Verification items for the finished model (mm, model axes). Face numbers are marked on the shaded views. A direction names the side the tool comes from. Coordinates: 2 decimals unless noted, no trailing zeros. Write each loop counter-clockwise with the first axis right and the second up, starting at its lowest first coordinate (ties: lowest second). Pieces come first, ordered by that corner, then holes. Notation, with made-up numbers: (22.5, 53) -> (62.5, 53) arc R10 cw to (62.5, 61) -> close; hole circle Ø1 at (7, -12.5). An arc over 180 degrees is marked (long way). Use CSV: the item, a comma, the result in double quotes.
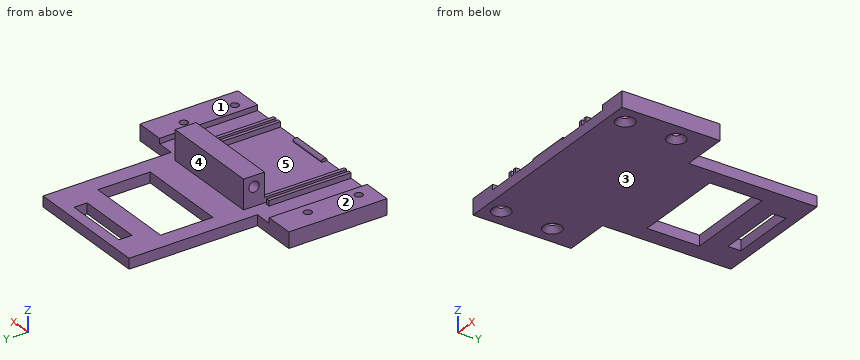
Solid Edge part; units mm, degrees
sketch "Sketch1" plane through (0, 0, 0) normal (0, 0, 1) x (1, 0, 0)
  line L0 (83.1, 37.5) -> (65.55, 37.5)
  line L1 (65.55, 37.5) -> (65.55, 86.5)
  line L2 (65.55, 86.5) -> (17.55, 86.5)
  line L3 (17.55, 86.5) -> (17.55, 37.5)
  line L4 (0, 37.5) -> (17.55, 37.5)
  line L5 (0, 0) -> (0, 37.5)
  line L6 (0, 0) -> (83.1, 0)
  line L7 (83.1, 0) -> (83.1, 37.5)
extrude "Protrusion1" add sketch "Sketch1" along normal blind 4
sketch "Sketch2" plane through (40.5, 43.25, 4) normal (0, 0, 1) x (1, 0, 0)
  line L0 (-29.5, -5.75) -> (-29.5, -43.25)
  line L1 (-29.5, -43.25) -> (-40.5, -43.25)
  line L2 (-40.5, -43.25) -> (-40.5, -5.75)
  line L3 (-40.5, -5.75) -> (-29.5, -5.75)
  line L4 (-20.53, -43.25) -> (-20.53, -11.85)
  line L5 (-20.53, -11.85) -> (-19.23, -11.85)
  line L6 (-19.23, -11.85) -> (-19.23, -43.25)
  line L7 (-19.23, -43.25) -> (-20.53, -43.25)
  line L8 (-16.73, -11.85) -> (-16.73, -43.25)
  line L9 (-16.73, -43.25) -> (-18.03, -43.25)
  line L10 (-18.03, -43.25) -> (-18.03, -11.85)
  line L11 (-18.03, -11.85) -> (-16.73, -11.85)
  line L12 (18.83, -11.85) -> (18.83, -43.25)
  line L13 (18.83, -43.25) -> (20.13, -43.25)
  line L14 (20.13, -43.25) -> (20.13, -11.85)
  line L15 (20.13, -11.85) -> (18.83, -11.85)
  line L16 (22.63, -43.25) -> (22.63, -11.85)
  line L17 (22.63, -11.85) -> (21.33, -11.85)
  line L18 (21.33, -11.85) -> (21.33, -43.25)
  line L19 (21.33, -43.25) -> (22.63, -43.25)
  line L20 (31.6, -5.75) -> (31.6, -43.25)
  line L21 (31.6, -43.25) -> (42.6, -43.25)
  line L22 (42.6, -43.25) -> (42.6, -5.75)
  line L23 (42.6, -5.75) -> (31.6, -5.75)
extrude "ExtrudedProtrusion_2" add sketch "Sketch2" along normal blind 2
sketch "Sketch3" plane through (41.55, 43.25, 4) normal (0, 0, 1) x (1, 0, 0)
  line L0 (-19.08, -11.85) -> (19.08, -11.85)
  line L1 (19.08, -11.85) -> (19.08, -3.85)
  line L2 (19.08, -3.85) -> (-19.08, -3.85)
  line L3 (-19.08, -3.85) -> (-19.08, -11.85)
extrude "ExtrudedProtrusion_3" add sketch "Sketch3" along normal blind 11.2
hole "Hole_1" at (60.63, 35.4, 11.2) direction (-1, 0, 0) diameter 4 depth 6
hole "Hole_2" at (22.47, 35.4, 11.2) direction (1, 0, 0) diameter 4 depth 6
sketch "Sketch4" plane through (41.55, 43.25, 4) normal (0, 0, 1) x (1, 0, 0)
  line L0 (12.5, 34.25) -> (-12.5, 34.25)
  line L1 (-12.5, 34.25) -> (-12.5, 39.25)
  line L2 (-12.5, 39.25) -> (12.5, 39.25)
  line L3 (12.5, 39.25) -> (12.5, 34.25)
  line L4 (-17.5, 26.75) -> (17.5, 26.75)
  line L5 (17.5, 26.75) -> (17.5, 6.75)
  line L6 (17.5, 6.75) -> (-17.5, 6.75)
  line L7 (-17.5, 6.75) -> (-17.5, 26.75)
extrude "Cutout1" cut sketch "Sketch4" against normal through all
hole "Hole_3" at (7, 6, 0) direction (0, 0, 1) diameter 3 end through all countersink diameter 6.94 countersink angle 90
hole "Hole1" at (7, 25.5, 0) direction (0, 0, 1) diameter 3 end through all countersink diameter 6.94 countersink angle 90
hole "Hole2" at (76.1, 6, 0) direction (0, 0, 1) diameter 3 end through all countersink diameter 6.94 countersink angle 90
hole "Hole3" at (76.1, 25.5, 0) direction (0, 0, 1) diameter 3 end through all countersink diameter 6.94 countersink angle 90
sketch "Sketch5" plane through (41.55, 15.7, 4) normal (0, 0, 1) x (1, 0, 0)
  line L0 (-8.0007, -13.7) -> (7.9993, -13.7)
  line L1 (7.9993, -13.7) -> (7.9993, -15.7)
  line L2 (-8.0007, -15.7) -> (7.9993, -15.7)
  line L3 (-8.0007, -13.7) -> (-8.0007, -15.7)
extrude "ExtrudedProtrusion_4" add sketch "Sketch5" along normal blind 1
fillet "Round_1" radius 0.6 2 edges at (41.5493, 2, 5) (41.5493, 0, 5)
1) Scan lines: L1, parallel to Y at x = 76.1, z = 4.35; L2, parallel to X at y = 24.5, z = 2; L3, parallel to Z at x = 56.8, y = 35.4. Record each from-to range of solid material in increasing order.
Return value:
L1,"0 to 4.5, 7.5 to 24, 27 to 37.5"
L2,"0 to 5.88, 8.12 to 74.98, 77.22 to 83.1"
L3,"0 to 9.2, 13.2 to 15.2"
2) Cross-section at D-D (y = 35.4). Record the boundary of the cut face in (x, z).
Return value:
outline,"(0, 0) -> (83.1, 0) -> (83.1, 6) -> (72.1, 6) -> (72.1, 4) -> (60.63, 4) -> (60.63, 9.2) -> (54.63, 9.2) -> (54.63, 13.2) -> (60.63, 13.2) -> (60.63, 15.2) -> (22.47, 15.2) -> (22.47, 13.2) -> (28.47, 13.2) -> (28.47, 9.2) -> (22.47, 9.2) -> (22.47, 4) -> (11, 4) -> (11, 6) -> (0, 6) -> close"
3) Mould release check, pull along X, two halves, no side actions. Record for the marked faces 4 and 5: released by +X, released by -X, zero draft, split by the parting line, or undercut.
Return value:
face 4,"zero draft"
face 5,"undercut"
4) Cross-section at B-B (y = 56). Record the boundary of the cut face in (x, z), plus the area to 3 significant figures.
Return value:
outline,"(17.55, 0) -> (24.05, 0) -> (24.05, 4) -> (17.55, 4) -> close; (59.05, 0) -> (65.55, 0) -> (65.55, 4) -> (59.05, 4) -> close"
area,"52.0 mm2"
5) Cross-section at C-C (x = 7). Record the boundary of the cut face in (y, z), plus the area to 3 significant figures.
Return value:
outline,"(0, 0) -> (2.53, 0) -> (4.5, 1.97) -> (4.5, 6) -> (0, 6) -> close; (7.5, 1.97) -> (9.47, 0) -> (22.03, 0) -> (24, 1.97) -> (24, 6) -> (7.5, 6) -> close; (27, 1.97) -> (28.97, 0) -> (37.5, 0) -> (37.5, 6) -> (27, 6) -> close"
area,"181 mm2"
6) Gauge pin test, flat ends, axial feed: pin 1 (1.8 mm diameter, centred on x = 8, z = 4, fed in from +Y); pin 2 (4.5 mm diameter, centred on y = 35.4, z = 11.2, fed in from +X); pin 3 (1 mm diameter, centred on x = 23, y = 16, fed in from +Z). Record the tip position at first contact, or that the pin passes through.
Return value:
pin 1,"y = 37.5"
pin 2,"x = 60.63"
pin 3,"z = 6"
7) Set-up check for the marked faces 1, 2 and 3: record each of +Z, -Z, +X, -X, +Y, -Y from which the full face is reachable in a straight line by a thin tool's end or side.
Return value:
face 1,"+Z, +X, +Y, -Y"
face 2,"+Z, -X, +Y, -Y"
face 3,"-Z, +X, -X, +Y, -Y"
8) Cross-section at A-A (x = 56.5). Record the boundary of the cut face in (y, z).
Return value:
outline,"(0, 0) -> (50, 0) -> (50, 4) -> (39.4, 4) -> (39.4, 15.2) -> (31.4, 15.2) -> (31.4, 4) -> (0, 4) -> close; (70, 0) -> (86.5, 0) -> (86.5, 4) -> (70, 4) -> close; hole circle Ø4 at (35.4, 11.2)"
